Input: part model. Units: mm. Frame: model coordinates. A direction names the side the tool comes from. Coordinates: 2 decimals unless noted, no trailing zeros. Write each loop counter-clockwise with the first axis right and the second up, starting at its lowest first coordinate (ties: lowest second). Pieces come first, ordered by that corner, then holes. Notation, with made-up numbers: (32, 41.25) -> (60, 41.25) arc R9 cw to (60, 55.25) -> close; hole circle Ø9 at (69, -24). An arc over 180 degrees is marked (long way). Use one line per item in the form item = value. Start each with the question number.
(1) Cut plane A-A on z = -27. Return the cut outline in (x, y).
(2) Cut plane C-C on x = 46.04. Return the cut outline in (y, z) (3 decimals), plus the area to 3 significant figures.
(3) Cut plane B-B on y = 15.5. Return the cut outline in (x, z).
(4) Cut plane D-D on z = -14. Return the cut outline in (x, y).
(5) Set-up query: faces 4 (the face through (9.28, 0.81, -2.32)), 5 (the face through (26, 1.59, -19)), 6 (the face through (0.81, 6.76, -18.94)). Return all of +Z, -Z, +X, -X, +Y, -Y with unobstructed straight access to the full face (end or side cutting, diameter ignored); none if empty.
(6) Pull-direction query (Y, two-part tool) for faces 1 (the face through (50.2, 0.81, -37.02)), 2 (the face through (26, 0, -19)), 3 (the face through (0.81, 18.8, -33.94)); classes: released by +Y, released by -Y, zero draft, split by the parting line, or undercut.
(7) First-contact query: pin 1 (4 mm diameter, centred on y = 24.5, z = -33.5, fed in from +X); pin 2 (3.5 mm diameter, centred on x = 7.94, z = -3.175, fed in from +Y); pin 3 (0.5 mm diameter, centred on x = 0.5, y = 21, fed in from -Z). Flat tips, straight axial feed; report the tip coordinate or a pass-through.
(8) Ray query, line 1 along Z through (x, y) = (46, 1); line 2 along Y through (x, z) = (19, -14). Return the intervals inside material, ascending.
```python
from build123d import *

# Parameters (mm, degrees)
ESQUISSE1_W             = 50.8
ESQUISSE1_H             = 37.59
BOSS_EXTRU_1_DEPTH      = 1.59
ESQUISSE2_W             = 1.59
ESQUISSE2_H             = 37.59
BOSS_EXTRU_2_DEPTH      = 37.59
CONG_1_R                = 1
ESQUISSE3_R             = 1.59
ENL_V_MAT_EXTRU_1_DEPTH = 74.52996804
CONG_2_R                = 2
ENL_V_MAT_EXTRU_2_DEPTH = 74.278268266
ESQUISSE5_R             = 1.625
ENL_V_MAT_EXTRU_3_DEPTH = 74.278268266


with BuildPart() as part:
    # Esquisse1 → Boss.-Extru.1 (new body)
    with BuildSketch(Plane(origin=(0, 0, 0), x_dir=(1, 0, 0), z_dir=(0, 1, 0))):
        with Locations((25.4, 18.795)):
            Rectangle(ESQUISSE1_W, ESQUISSE1_H)
    extrude(amount=BOSS_EXTRU_1_DEPTH)

    # Esquisse2 → Boss.-Extru.2 (add)
    with BuildSketch(Plane(origin=(0, 1.59, 0), x_dir=(-1, 0, 0), z_dir=(0, 1, 0))):
        with Locations((-0.795, -18.795)):
            Rectangle(ESQUISSE2_W, ESQUISSE2_H)
    extrude(amount=BOSS_EXTRU_2_DEPTH)

    # Congé1
    cong_1_edges = [part.edges().sort_by_distance(p)[0] for p in [
        (0, 0, -18.795),
    ]]
    fillet(cong_1_edges, radius=CONG_1_R)

    # Esquisse3 → Enlèv. mat.-Extru.1 (cut, through all)
    with BuildSketch(Plane(origin=(0, 1.59, 0), x_dir=(1, 0, 0), z_dir=(0, 1, 0))):
        with Locations(Location((7.94, 34.415, 0), (0, 0, 270))):
            Circle(ESQUISSE3_R)
        with Locations(Location((14.29, 34.415, 0), (0, 0, 270))):
            Circle(ESQUISSE3_R)
        with Locations(Location((20.64, 34.415, 0), (0, 0, 270))):
            Circle(ESQUISSE3_R)
        with Locations(Location((26.99, 34.415, 0), (0, 0, 270))):
            Circle(ESQUISSE3_R)
        with Locations(Location((33.34, 34.415, 0), (0, 0, 270))):
            Circle(ESQUISSE3_R)
        with Locations(Location((39.69, 34.415, 0), (0, 0, 270))):
            Circle(ESQUISSE3_R)
        with Locations(Location((46.04, 34.415, 0), (0, 0, 270))):
            Circle(ESQUISSE3_R)
        with Locations(Location((46.04, 3.175, 0), (0, 0, 270))):
            Circle(ESQUISSE3_R)
        with Locations(Location((39.69, 3.175, 0), (0, 0, 270))):
            Circle(ESQUISSE3_R)
        with Locations(Location((33.34, 3.175, 0), (0, 0, 270))):
            Circle(ESQUISSE3_R)
        with Locations(Location((26.99, 3.175, 0), (0, 0, 270))):
            Circle(ESQUISSE3_R)
        with Locations(Location((20.64, 3.175, 0), (0, 0, 270))):
            Circle(ESQUISSE3_R)
        with Locations(Location((14.29, 3.175, 0), (0, 0, 270))):
            Circle(ESQUISSE3_R)
        with Locations(Location((7.94, 3.175, 0), (0, 0, 270))):
            Circle(ESQUISSE3_R)
    extrude(amount=-ENL_V_MAT_EXTRU_1_DEPTH, mode=Mode.SUBTRACT)

    # Congé2
    cong_2_edges = [part.edges().sort_by_distance(p)[0] for p in [
        (50.8, 0.795, 0),
        (50.8, 0.795, -37.59),
    ]]
    fillet(cong_2_edges, radius=CONG_2_R)

    # Esquisse4 → Enlèv. mat.-Extru.2 (cut, through all)
    with BuildSketch(Plane(origin=(1.59, 0, 0), x_dir=(0, 0, -1), z_dir=(1, 0, 0))):
        with BuildLine():
            Line((0, 39.18), (0, 20.385))
            ThreePointArc((0, 20.385), (5.504928048, 33.675071952), (18.795, 39.18))
            Line((18.795, 39.18), (0, 39.18))
        make_face()
        with BuildLine():
            Line((37.59, 39.18), (18.795, 39.18))
            ThreePointArc((18.795, 39.18), (32.085071952, 33.675071952), (37.59, 20.385))
            Line((37.59, 20.385), (37.59, 39.18))
        make_face()
    extrude(amount=-ENL_V_MAT_EXTRU_2_DEPTH, mode=Mode.SUBTRACT)

    # Esquisse5 → Enlèv. mat.-Extru.3 (cut, through all)
    with BuildSketch(Plane(origin=(1.59, 0, 0), x_dir=(0, 0, -1), z_dir=(1, 0, 0))):
        with Locations((34.295, 20.385)):
            Circle(ESQUISSE5_R)
        with Locations((26.545, 6.961606241)):
            Circle(ESQUISSE5_R)
        with Locations((11.045, 6.961606241)):
            Circle(ESQUISSE5_R)
        with Locations((3.295, 20.385)):
            Circle(ESQUISSE5_R)
        with Locations((11.045, 33.808393759)):
            Circle(ESQUISSE5_R)
        with Locations((26.545, 33.808393759)):
            Circle(ESQUISSE5_R)
        with BuildLine():
            Line((12.19, 13.365), (12.19, 27.405))
            ThreePointArc((12.19, 27.405), (18.795, 34.01), (25.4, 27.405))
            Line((25.4, 27.405), (25.4, 13.365))
            ThreePointArc((25.4, 13.365), (18.795, 6.76), (12.19, 13.365))
        make_face()
    extrude(amount=-ENL_V_MAT_EXTRU_3_DEPTH, mode=Mode.SUBTRACT)


solid = part.part
```
Values:
q1.outline = (0, 1) arc R1 ccw to (1, 0) -> (50.8, 0) -> (50.8, 1.59) -> (1.59, 1.59) -> (1.59, 5.4) -> (0, 5.4) -> close; (0, 8.52) -> (1.59, 8.52) -> (1.59, 32.25) -> (0, 32.25) -> close; (0, 35.37) -> (1.59, 35.37) -> (1.59, 37.29) -> (0, 37.29) -> close
q2.outline = (0, -37.59) -> (1.59, -37.59) -> (1.59, -36.005) -> (0, -36.005) -> close; (0, -32.825) -> (1.59, -32.825) -> (1.59, -4.765) -> (0, -4.765) -> close; (0, -1.585) -> (1.59, -1.585) -> (1.59, 0) -> (0, 0) -> close
q2.area = 49.7 mm2
q3.outline = (0, -37.59) -> (1.59, -37.59) -> (1.59, -25.4) -> (0, -25.4) -> close; (0, -12.19) -> (1.59, -12.19) -> (1.59, 0) -> (0, 0) -> close
q4.outline = (0, 1) arc R1 ccw to (1, 0) -> (50.8, 0) -> (50.8, 1.59) -> (1.59, 1.59) -> (1.59, 8.82) -> (0, 8.82) -> close; (0, 31.95) -> (1.59, 31.95) -> (1.59, 38.56) -> (0, 38.56) -> close
q5.face_4 = +Y, -Y
q5.face_5 = +Z, -Z, +X, +Y
q5.face_6 = +X, -X
q6.face_1 = zero draft
q6.face_2 = released by -Y
q6.face_3 = undercut
q7.pin_1 = 1.59
q7.pin_2 = 1.59
q7.pin_3 = -37.59
q8.line_1 = -37.59 to -36, -32.83 to -4.76, -1.59 to 0
q8.line_2 = 0 to 1.59
